Could you check a few things on this model? Use its own coordinates, in mm. Face numbers are marked on the shaded views. Give positions to 0.01 mm unless a question says otherwise; leave off trailing zeros. Loops run counter-clockwise (first coordinate to the right, second up) from the corner with the lowest first, then second, coordinate; pieces in that order, holes last. Notation, with made-up numbers: M 89.25,74 L 126.25,74 A21 ccw 126.25,94 Z; hole C 5,8 d8. An arc over 180 degrees is marked long. Return JSON: item names as keys, results as strings. Group by question number.
1. If we mould it in two halves opening along X, with no side actions, what happens to the marked faces 1, 2 and 3? For each: +X half, -X half, draft (parallel to the pull), parting line (faces both ways), or undercut.
2. If we section it at C-C (z = 16): Write out the boundary of the cut face in (x, y), plus the area to 3 significant figures.
3. Please list where these lines run through material, in increasing order: line 1 (Y direction, x = 0, z = 19.5); line 2 (X direction, y = 0.5, z = 2); line 3 (X direction, y = -11.5, z = 15.5).
4. For pin 1 (1.5 mm diameter, centred on x = 13.5, z = 24.5, fed in from +Y); pin 2 (5 mm diameter, centred on y = -4.5, z = 20, fed in from +X); pin 3 (4 mm diameter, centred on x = 4, z = 23.5, fed in from +Y); pin 4 (12 mm diameter, centred on y = 0.5, z = 13.5, fed in from +X), each with a flat end and sliding along its axis, tell me the tip position at first contact or that it passes through.
5. If we section it at A-A (x = 0): Write out the boundary of the cut face in (y, z), plus the area to 3 significant figures.
6. If we section it at B-B (z = 5): Write out the boundary of the cut face in (x, y), plus the area to 3 significant figures.
```python
from build123d import *

# Parameters (mm, degrees)
F0_R     = 17.25
F0_R_2   = 14.45
F1_DEPTH = 33
F0_R_3   = 19.1
F2_DEPTH = 8.3
F3_R     = 1


with BuildPart() as f1:
    # F0 (on Top) → F1 (new body)
    with BuildSketch(Plane.XY):
        Circle(F0_R)
        Circle(F0_R_2, mode=Mode.SUBTRACT)
    extrude(amount=F1_DEPTH)

    # F0 (on Top) → F2 (join)
    with BuildSketch(Plane.XY):
        Circle(F0_R_3)
        Circle(F0_R, mode=Mode.SUBTRACT)
    extrude(amount=F2_DEPTH)

    # F3
    f3_edges = [f1.edges().sort_by_distance(p)[0] for p in [
        (-17.25, 0, 33),
        (-14.45, 0, 33),
    ]]
    fillet(f3_edges, radius=F3_R)


solid = f1.part
```
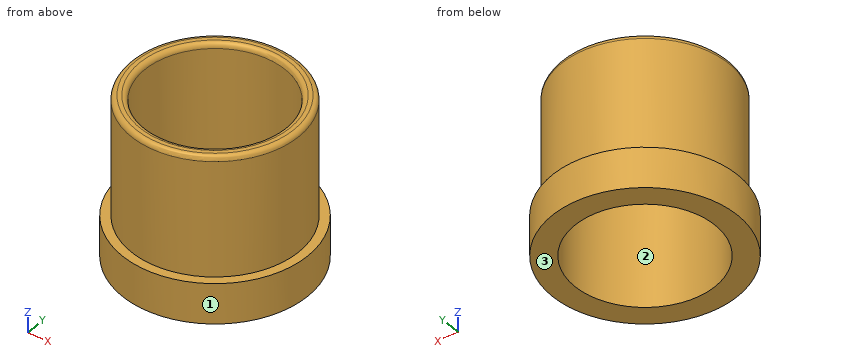
Answer:
{
 "1": {"face 1": "parting line", "face 2": "undercut", "face 3": "draft"},
 "2": {"outline": "C 0,0 d34.5; hole C 0,0 d28.9", "area": "279 mm²"},
 "3": {"line 1": "y = -17.25 to -14.45, 14.45 to 17.25", "line 2": "x = -19.09 to -14.44, 14.44 to 19.09", "line 3": "x = -12.86 to -8.75, 8.75 to 12.86"},
 "4": {"pin 1": "stops at y = 11.62", "pin 2": "stops at x = 17.13", "pin 3": "stops at y = 17.13", "pin 4": "stops at x = 19.1"},
 "5": {"outline": "M -19.1,0 L -14.45,0 L -14.45,32 A1 ccw -15.45,33 L -16.25,33 A1 ccw -17.25,32 L -17.25,8.3 L -19.1,8.3 Z; M 14.45,0 L 19.1,0 L 19.1,8.3 L 17.25,8.3 L 17.25,32 A1 ccw 16.25,33 L 15.45,33 A1 ccw 14.45,32 Z", "area": "215 mm²"},
 "6": {"outline": "C 0,0 d38.2; hole C 0,0 d28.9", "area": "490 mm²"}
}
